Build history of the part. All positions in model axes, mm. A direction names the side the tool comes from. Round coordinates to 2 decimals unless told otherwise and drop trailing zeros. Loops run counter-clockwise (first coordinate to the right, second up) from the corner with the lowest first, then second, coordinate; pieces in that order, holes last. Notation, with made-up numbers: M -5,58 L 27,58 A9 ccw 27,62 Z; hole C 51,43 d2. An arc over 180 degrees is marked long. One line per item, written item: value.
```python
from build123d import *

# Parameters (mm, degrees)
F0_R     = 1.5
F1_DEPTH = 3
F3_DEPTH = 10
F4_DEPTH = 10.001


with BuildPart() as f1:
    # F0 (on Top) → F1 (new body)
    with BuildSketch(Plane.XY):
        with BuildLine():
            Line((-5, -17.5), (5, -17.5))
            Line((5, -17.5), (5, 17.5))
            ThreePointArc((5, 17.5), (0, 22.5), (-5, 17.5))
            Line((-5, 17.5), (-5, -17.5))
        make_face()
        with Locations((0, 17.5)):
            Circle(F0_R, mode=Mode.SUBTRACT)
    extrude(amount=F1_DEPTH)

    # F2 (on face) → F3 (join, through all)
    with BuildSketch(Plane(origin=(-5, 0, 0), x_dir=(0, -1, 0), z_dir=(-1, 0, 0))):
        with BuildLine():
            ThreePointArc((15, 3), (16.0606601718, 2.5606601718), (16.5, 1.5))
            ThreePointArc((16.5, 1.5), (16.0606601718, 0.4393398282), (15, 0))
            Line((15, 0), (17.5, 0))
            Line((17.5, 0), (17.5, 3))
            Line((17.5, 3), (15, 3))
        make_face()
        with BuildLine():
            Line((12.4019237886, 3), (15, 3))
            Line((15, 3), (17.5, 3))
            Line((17.5, 3), (17.5, 0))
            Line((17.5, 0), (15, 0))
            Line((15, 0), (12.4019237886, 0))
            ThreePointArc((12.4019237886, 0), (15.7764571353, -1.3977774789), (18, 1.5))
            ThreePointArc((18, 1.5), (15.7764571353, 4.3977774789), (12.4019237886, 3))
        make_face()
    extrude(amount=-F3_DEPTH)

    # F2 (on face) → F4 (cut, through all)
    with BuildSketch(Plane(origin=(-5, 0, 0), x_dir=(0, -1, 0), z_dir=(-1, 0, 0))):
        with BuildLine():
            ThreePointArc((15, 0), (16.0606601718, 0.4393398282), (16.5, 1.5))
            ThreePointArc((16.5, 1.5), (16.0606601718, 2.5606601718), (15, 3))
            ThreePointArc((15, 3), (13.5, 1.5), (15, 0))
        make_face()
    extrude(amount=-F4_DEPTH, mode=Mode.SUBTRACT)


solid = f1.part
```
Item 1: Slice it at C-C, the plane y = 16.5. Give the cut face in (x, z).
Check values:
outline: M -5,0 L -1.12,0 L -1.12,3 L -5,3 Z; M 1.12,0 L 5,0 L 5,3 L 1.12,3 Z
Item 2: Slice it at A-A, the plane x = 0. Give the cut face in (y, z).
Check values:
outline: M -12.4,0 L 16,0 L 16,3 L -12.4,3 A3 ccw long Z; M 19,0 L 22.5,0 L 22.5,3 L 19,3 Z; hole C -15,1.5 d3
Item 3: Which spindle directions (+Z, -Z, +X, -X, +Y, -Y) get a long thin tool onto all of the face, cutting with end or side? Do faces 4 (the face through (0, 5, 0)), 5 (the face through (5, 0, 2)). Say none if no direction does.
Check values:
face 4: -Z, +X, -X, +Y
face 5: +Z, -Z, +X, +Y, -Y
Item 4: Wall check: line 1 along Y through (x, z) = (0, 1.75); line 2 along Y through (x, z) = (0, 0.8); line 3 along Z through (x, y) = (3.75, -12). Give the ranges that are in metal, low to high.
Check values:
line 1: y = -17.99 to -16.48, -13.52 to 16, 19 to 22.5
line 2: y = -17.92 to -16.33, -13.67 to 16, 19 to 22.5
line 3: z = 0 to 3
Item 5: Slice it at D-D, the plane x = 2.75. Give the cut face in (y, z), and give its area (3 significant figures).
Check values:
outline: M -12.4,0 L 21.68,0 L 21.68,3 L -12.4,3 A3 ccw long Z; hole C -15,1.5 d3
area: 123 mm2
Item 6: Drop flat-ended pins along their axis: P1, Ø3, axis at x = 1.5, y = 9, coming from the -Z side; P2, Ø1.5, axis at x = 3.5, z = 0.5, coming from the +Y side; P3, Ø1, axis at x = 3.5, y = 1, coming from the +Z side. Give the stop position or say it passes through.
Check values:
P1: stops at z = 0
P2: stops at y = 21.68
P3: stops at z = 3
Item 7: Pull direction X, two halves, no side cores. Call faces 1 (the face through (0, 19, 1)), 2 (the face through (-5, 0, 1)), 3 (the face through (0, 5, 3)): pulls with the +X half, pulls with the -X half, needs draft (parallel to the pull), parting line crosses it, or undercut.
Check values:
face 1: undercut
face 2: pulls with the -X half
face 3: needs draft
Item 8: Slice it at B-B, the plane z = 2. Give the cut face in (x, y).
Check values:
outline: M -5,-17.96 L 5,-17.96 L 5,-16.41 L -5,-16.41 Z; M -5,-13.59 L 5,-13.59 L 5,17.5 A5 ccw -5,17.5 Z; hole C 0,17.5 d3
